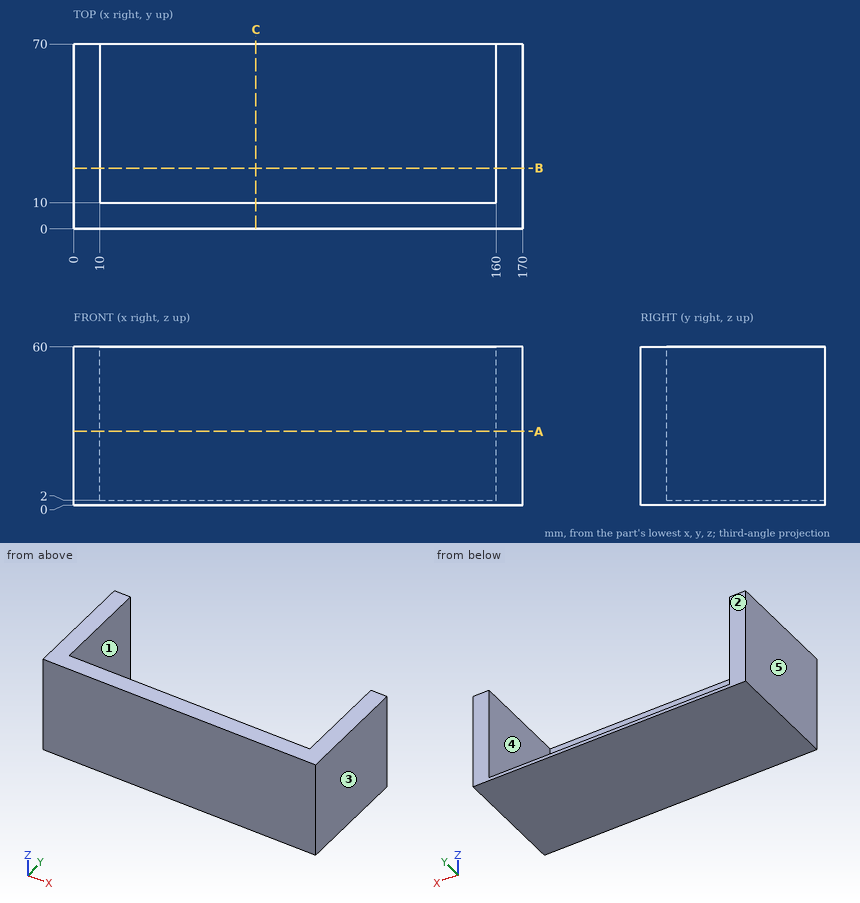
Part print with two shaded views. Sizes in mm from the minimum x, y, z corner. A direction names the side the tool comes from. Round coordinates to 2 decimals unless told otherwise and drop trailing zeros. Order: outer loops, then holes, each group sorted by start corner. A loop starts at its lowest first (then second) coordinate and runs counter-clockwise, first axis right, second up. Notation, with made-up numbers: M -32,-17 L 12,-17 A24 ccw 12,17 Z; hole C -22.75,9 d9. An arc over 180 degrees is marked long. Answer in a Markdown table with one row per item. Add a question column.
Q1. Wall check: L1, parallel to X at y = 67, z = 36.5; L2, parallel to Y at x = 155.5, z = 37; L3, parallel to Z at x = 107, y = 43. Give the ranges that are in metal, low to high. Write a range as from..to.
Q2. 3-axis set-ups, long thin cutter, end or side, ignore diameter. For the marked faces 1 and 2: which of +Z, -Z, +X, -X, +Y, -Y reach the whole face in a straight line?
Q3. Cut at C-C on x = 69. Give the cut face in (y, z), and give its area (3 significant figures).
Q4. Pin check, flat tips, straight feed: pin 1 (12 mm diameter, centred on x = 139, y = 51, fed in from +Z); pin 2 (1.5 mm diameter, centred on x = 107, z = 47.5, fed in from +Y). Stop position of each tip, or through.
Q5. Cut at A-A on z = 28. Give the cut face in (x, y), and give its area (3 significant figures).
Q6. Cut at B-B on y = 23. Give the cut face in (x, z), and give its area (3 significant figures).
Q7. Mould opens along X. For the marked faces 3, 4 and 5 say: +X half, -X half, draft (parallel to the pull), parting line (faces both ways), or undercut.
Established:
| question | item | result |
|---|---|---|
| 1 | L1 | x = 0..10, 160..170 |
| 1 | L2 | y = 0..10 |
| 1 | L3 | z = 0..2 |
| 2 | face 1 | +Z, +Y |
| 2 | face 2 | +Z, -Z, +X, -X, +Y |
| 3 | outline | M 0,0 L 70,0 L 70,2 L 10,2 L 10,60 L 0,60 Z |
| 3 | area | 720 mm2 |
| 4 | pin 1 | stops at z = 2 |
| 4 | pin 2 | stops at y = 10 |
| 5 | outline | M 0,0 L 170,0 L 170,70 L 160,70 L 160,10 L 10,10 L 10,70 L 0,70 Z |
| 5 | area | 2,900 mm2 |
| 6 | outline | M 0,0 L 170,0 L 170,60 L 160,60 L 160,2 L 10,2 L 10,60 L 0,60 Z |
| 6 | area | 1,500 mm2 |
| 7 | face 3 | +X half |
| 7 | face 4 | undercut |
| 7 | face 5 | -X half |
